Work out the finished part from the listing and answer in its coordinate system (mm). Round coordinates to 2 decimals unless told otherwise and drop trailing zeros. Write each loop counter-clockwise with the first axis right and the second up, starting at its lowest first coordinate (ties: lowest second). Pieces come first, ordered by that corner, then holes.
1. Flat-ended cylindrical pins translate along their axes: pin 1 Ø18 at (x, z) = (-101.18, 232.01) entering from +Y; pin 2 Ø2 at (x, y) = (-105, 289.5) entering from -Z; pin 3 Ø2 at (x, y) = (-102, 289.5) entering from +Z; pin 4 Ø1 at (y, z) = (290, 178) entering from -X. Find the tip coordinate at first contact, or state that the pin passes through.
2. Find section C-C (x = -101). Write down the section's boundary in (y, z), and give its area (3 significant figures).
3. Find section B-B (z = 225). Write down the section's boundary in (x, y), and give its area (3 significant figures).
4. Straight lines are drawn through the part: probe 1 along Z at (x, y) = (-101, 290.05); probe 2 along Z at (x, y) = (-42.5, 289.25); probe 3 along Z at (x, y) = (-64, 291.2). For each, find the intervals that lie inside material, in ascending order.
5. Find section D-D (y = 288.95). Count the separate pieces of the cut face and the enclosed holes in it, and give its area (3 significant figures).
6. Find section A-A (x = -49). Write down the section's boundary in (y, z).
Autodesk Inventor part; units mm, degrees
ref_plane "РабПлоскость2" through (-105.2734, 252.5455, 159.0129) normal (-1, 0, 0) x (0, 0, 1)
ref_plane "YZ Plane" through (0, 0, 0) normal (1, 0, 0) x (0, 1, 0)
ref_plane "XZ Plane" through (0, 0, 0) normal (0, 1, 0) x (-1, 0, 0)
ref_plane "РабПлоскость1" through (-53.4845, 288.2505, 354.5129) normal (0, 1, 0) x (-1, 0, 0)
sketch "Эскиз1" plane through (-53.4845, 288.2505, 354.5129) normal (0, 1, 0) x (-1, 0, 0)
  line L0 (45.7889, -56.5016) -> (45.7889, -62.7516)
  line L1 (-13.3, 2.5) -> (-13.3, -247.5)
  line L2 (-13.3, -220) -> (32.7, -220)
  line L3 (32.7, -220) -> (32.7, -25)
  line L4 (32.7, -25) -> (-13.3, -25)
  line L5 (-13.3, -25) -> (-13.3, -220)
  line L6 (-5.3, -220) -> (142.8907, -220)
  line L7 (201.7, -25) -> (166.8907, -25)
  point P0 (-53.4845, -354.5129)
  point P1 (-13.3, -25)
  point P2 (-13.3, -220)
  point P3 (32.7, -62.75)
  point P4 (32.7, -56.5)
extrude "Выдавливание1" add sketch "Эскиз1" along normal blind 4
sketch "Эскиз6" plane through (-53.4845, 288.2505, 354.5129) normal (0, -1, 0) x (1, 0, 0)
  line L0 (-32.7, -169.6539) -> (-20.7, -169.6539)
  line L1 (-32.7, -175.6539) -> (-32.7, -169.6539)
  line L2 (-20.7, -175.6539) -> (-32.7, -175.6539)
  line L3 (-20.7, -175.6539) -> (-20.7, -169.6539)
  line L4 (-32.7, -69.3164) -> (-20.7, -69.3164)
  line L5 (-32.7, -75.3164) -> (-32.7, -69.3164)
  line L6 (-20.7, -75.3164) -> (-32.7, -75.3164)
  line L7 (-20.7, -75.3164) -> (-20.7, -69.3164)
  line L8 (13.3, -220) -> (-32.7, -220)
  line L9 (-9.7, -220) -> (-9.7, 17.4543)
  line L10 (13.3, -169.6539) -> (1.3, -169.6539)
  line L11 (13.3, -175.6539) -> (13.3, -169.6539)
  line L12 (1.3, -175.6539) -> (13.3, -175.6539)
  line L13 (1.3, -175.6539) -> (1.3, -169.6539)
  line L14 (13.3, -69.3164) -> (1.3, -69.3164)
  line L15 (13.3, -75.3164) -> (13.3, -69.3164)
  line L16 (1.3, -75.3164) -> (13.3, -75.3164)
  line L17 (1.3, -75.3164) -> (1.3, -69.3164)
  point P0 (53.4845, -354.5129)
extrude "Выдавливание3" cut sketch "Эскиз6" against normal blind 8
sketch "Эскиз7" plane through (-53.4845, 288.2505, 354.5129) normal (0, -1, 0) x (1, 0, 0)
  line L0 (-12.95, -175.6539) -> (-12.95, -169.6539)
  line L1 (-7.95, -169.6539) -> (-7.95, -175.6539)
  line L2 (-6.45, -175.6539) -> (-6.45, -169.6539)
  line L3 (-11.45, -175.6539) -> (-11.45, -169.6539)
  line L4 (-12.95, -175.6539) -> (-12.95, -169.6539)
  line L5 (-11.45, -175.6539) -> (-7.95, -175.6539)
  line L6 (-7.95, -175.6539) -> (-7.95, -169.6539)
  line L7 (-7.95, -169.6539) -> (-11.45, -169.6539)
  line L8 (-11.45, -169.6539) -> (-11.45, -175.6539)
  circle A0 centre (-9.7, -172.6539) radius 1.75
  line L9 (-32.7, -122.4852) -> (36.9657, -122.4852)
  line L10 (-12.95, -69.3164) -> (-12.95, -75.3164)
  line L11 (-7.95, -75.3164) -> (-7.95, -69.3164)
  line L12 (-6.45, -69.3164) -> (-6.45, -75.3164)
  line L13 (-11.45, -69.3164) -> (-11.45, -75.3164)
  line L14 (-12.95, -69.3164) -> (-12.95, -75.3164)
  line L15 (-11.45, -69.3164) -> (-7.95, -69.3164)
  line L16 (-7.95, -69.3164) -> (-7.95, -75.3164)
  line L17 (-7.95, -75.3164) -> (-11.45, -75.3164)
  line L18 (-11.45, -75.3164) -> (-11.45, -69.3164)
  circle A1 centre (-9.7, -72.3164) radius 1.75
  point P0 (53.4845, -354.5129)
extrude "Выдавливание4" cut sketch "Эскиз7" against normal blind 8 contours A0 | A1
sketch "Эскиз8" plane through (-53.4845, 288.2505, 354.5129) normal (0, -1, 0) x (1, 0, 0)
  line L0 (-45.7889, -165.5) -> (-60.7889, -165.5)
  line L1 (-60.7889, -165.5) -> (-60.7889, -79.5)
  line L2 (-60.7889, -79.5) -> (-45.7889, -79.5)
  line L3 (-45.7889, -79.5) -> (-45.7889, -165.5)
  point P0 (53.4845, -354.5129)
  point P1 (-51.7889, -79.5)
  dimension "d15" = 15
extrude "Выдавливание5" add sketch "Эскиз8" against normal blind 4
sketch "Эскиз9" plane through (-53.4845, 288.2505, 354.5129) normal (0, -1, 0) x (1, 0, 0)
  circle A0 centre (-58.2, -138) radius 1.2645
  circle A1 centre (-58.2, -107) radius 1.2645
  circle A2 centre (-27.2, -107) radius 1.2645
  circle A3 centre (-27.2, -138) radius 1.2645
  point P0 (53.4845, -354.5129)
extrude "Выдавливание6" cut sketch "Эскиз9" against normal blind 4
sketch "Эскиз11" plane through (-86.1845, 288.2505, 329.5129) normal (-1, 0, 0) x (0, 0, 1)
  line L0 (-160.6539, 0) -> (-150.6539, 0)
  line L1 (-150.6539, 0) -> (-150.6539, 4)
  line L2 (-150.6539, 4) -> (-160.6539, 4)
  line L3 (-160.6539, 4) -> (-160.6539, 0)
  line L4 (-44.6539, 4) -> (-34.6539, 4)
  line L5 (-34.6539, 4) -> (-34.6539, 0)
  line L6 (-34.6539, 0) -> (-44.6539, 0)
  line L7 (-44.6539, 0) -> (-44.6539, 4)
  point P0 (-329.5129, -288.2505)
ref_plane "РабПлоскость2" through (-105.2734, 252.5455, 159.0129) normal (-1, 0, 0) x (0, 0, 1)
extrude "Выдавливание8" add sketch "Эскиз11" along normal up to surface (19.0889 mm away)
sketch "Эскиз12" plane through (-53.4845, 288.2505, 354.5129) normal (0, -1, 0) x (1, 0, 0)
  line L0 (-60.7889, -79.5) -> (-60.7889, -165.5)
  line L1 (-32.7, -220) -> (-32.7, -25)
  line L2 (-60.7889, -79.5) -> (-32.7, -79.5)
  line L3 (-32.7, -79.5) -> (-32.7, -165.5)
  line L4 (-32.7, -165.5) -> (-60.7889, -165.5)
  line L5 (-60.7889, -165.5) -> (-60.7889, -79.5)
  point P0 (53.4845, -354.5129)
  point P1 (-32.7, -169.6539)
  point P2 (-32.7, -75.3164)
  point P3 (-32.7, -185.6539)
  dimension "d24" = 86
extrude "Выдавливание9" add sketch "Эскиз12" against normal blind 4
sketch "Эскиз13" plane through (-53.4845, 288.2505, 354.5129) normal (0, -1, 0) x (1, 0, 0)
  circle A0 centre (-58.2, -107) radius 1.2645
  circle A1 centre (-58.2, -138) radius 1.2645
  circle A2 centre (-42.7, -122.5) radius 3.3
  point P0 (53.4845, -354.5129)
extrude "Выдавливание10" cut sketch "Эскиз13" against normal blind 8
sketch "Эскиз14" plane through (-53.4845, 288.2505, 354.5129) normal (0, -1, 0) x (1, 0, 0)
  line L0 (-45.7603, -165.5) -> (-45.7603, -175.6539)
  line L1 (-45.7603, -175.6539) -> (-32.7, -175.6539)
  line L2 (-45.7603, -185.6539) -> (-32.7, -185.6539)
  line L3 (-32.7, -185.6539) -> (-32.7, -220)
  line L4 (-32.7, -220) -> (-45.7603, -220)
  line L5 (-45.7603, -220) -> (-45.7603, -185.6539)
  line L6 (-45.7603, -79.5) -> (-45.7603, -69.6539)
  line L7 (-45.7603, -59.6539) -> (-45.7603, -25)
  line L8 (-45.7603, -25) -> (-32.7, -25)
  line L9 (-32.7, -79.5) -> (-45.7603, -79.5)
  line L10 (-45.7603, -79.5) -> (-45.7603, -69.6539)
  line L11 (-45.7603, -25) -> (-32.7, -25)
  line L12 (-32.7, -25) -> (-32.7, -59.6539)
  line L13 (-32.7, -59.6539) -> (-45.7603, -59.6539)
  line L14 (-45.7603, -59.6539) -> (-45.7603, -25)
  line L15 (-45.7603, -79.5) -> (-32.7, -79.5)
  line L16 (-32.7, -79.5) -> (-32.7, -69.6539)
  line L17 (-32.7, -69.6539) -> (-45.7603, -69.6539)
  line L18 (-45.7603, -69.6539) -> (-45.7603, -79.5)
  line L19 (-45.7603, -175.6539) -> (-32.7, -175.6539)
  line L20 (-32.7, -175.6539) -> (-32.7, -165.5)
  line L21 (-32.7, -165.5) -> (-45.7603, -165.5)
  line L22 (-45.7603, -165.5) -> (-45.7603, -175.6539)
  point P0 (53.4845, -354.5129)
  point P1 (13.3, -220)
  point P2 (-32.7, -25)
  point P3 (-45.7603, -69.6539)
  point P4 (-45.7603, -165.5)
extrude "Выдавливание11" add sketch "Эскиз14" against normal blind 4
sketch "Эскиз16" plane through (-53.4845, 288.2505, 354.5129) normal (0, -1, 0) x (1, 0, 0)
  circle A0 centre (-42.7, -122.5) radius 4.1
  circle A1 centre (-47.7, -122.5) radius 10
  circle A2 centre (-58.2, -107) radius 1.2645
  circle A3 centre (-27.2, -107) radius 1.2645
  circle A4 centre (-27.2, -138) radius 1.2645
  circle A5 centre (-58.2, -138) radius 1.2645
  circle A6 centre (-63.2, -107) radius 1.2645
  circle A7 centre (-32.2, -107) radius 1.2645
  circle A8 centre (-63.2, -138) radius 1.2645
  circle A9 centre (-32.2, -138) radius 1.2645
  point P0 (53.4845, -354.5129)
  dimension "d35" = 5
  dimension "d36" = 0
  dimension "d37" = 20
  dimension "d38" = 5
  dimension "d39" = 5
  dimension "d40" = 5
  dimension "d41" = 5
extrude "Выдавливание13" cut sketch "Эскиз16" against normal blind 10 contours A0 | A1 | A6 | A7 | A8 | A9
properties part number "крепление Y"
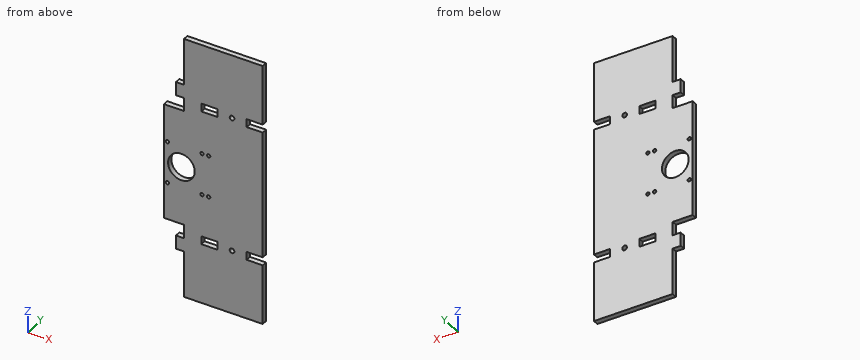
Worked answers:
1. pin 1: passes through
1. pin 2: stops at z = 168.86
1. pin 3: stops at z = 294.86
1. pin 4: stops at x = -105.27
2. outline: (288.25, 168.86) - (292.25, 168.86) - (292.25, 178.86) - (288.25, 178.86) - close; (288.25, 189.01) - (292.25, 189.01) - (292.25, 222.01) - (288.25, 222.01) - close; (288.25, 242.01) - (292.25, 242.01) - (292.25, 275.01) - (288.25, 275.01) - close; (288.25, 284.86) - (292.25, 284.86) - (292.25, 294.86) - (288.25, 294.86) - close
2. area: 344 mm2
3. outline: (-114.27, 288.25) - (-108.31, 288.25) - (-108.31, 292.25) - (-114.27, 292.25) - close; (-94.06, 288.25) - (-40.18, 288.25) - (-40.18, 292.25) - (-94.06, 292.25) - close
3. area: 239 mm2
4. probe 1: z = 168.86 to 178.86, 189.01 to 222.01, 242.01 to 275.01, 284.86 to 294.86
4. probe 2: z = 134.51 to 178.86, 184.86 to 279.2, 285.2 to 329.51
4. probe 3: z = 134.51 to 180.31, 183.41 to 280.65, 283.74 to 329.51
5. separate pieces: 1
5. enclosed holes: 11
5. area: 12,300 mm2
6. outline: (288.25, 134.51) - (292.25, 134.51) - (292.25, 178.86) - (288.25, 178.86) - close; (288.25, 184.86) - (292.25, 184.86) - (292.25, 279.2) - (288.25, 279.2) - close; (288.25, 285.2) - (292.25, 285.2) - (292.25, 329.51) - (288.25, 329.51) - close
